from build123d import *

# Parameters (mm, degrees)
SKETCH1_W           = 38.354
SKETCH1_H           = 44.45
BOSS_EXTRUDE1_DEPTH = 25.4
SKETCH2_R           = 3.429
CUT_EXTRUDE1_DEPTH  = 44.45
SKETCH3_R           = 1.7272
CUT_EXTRUDE2_DEPTH  = 12.7
SKETCH5_R           = 1.7272
CUT_EXTRUDE4_DEPTH  = 12.7
SKETCH6_R           = 3.429
CUT_EXTRUDE5_DEPTH  = 38.354
SKETCH7_R           = 1.7272
CUT_EXTRUDE6_DEPTH  = 9.525
SKETCH11_W          = 38.354
SKETCH11_H          = 12.954
CUT_EXTRUDE9_DEPTH  = 3.2512
CUT_EXTRUDE7_START  = -7.62
SKETCH8_R           = 1.7272
CUT_EXTRUDE7_DEPTH  = 7.62
BOSS_EXTRUDE2_START = 2.54
SKETCH9_R           = 1.7272
SKETCH9_R_2         = 3.429
BOSS_EXTRUDE2_DEPTH = 2.54
SKETCH12_W          = 13.97
SKETCH12_H          = 25.4
CUT_EXTRUDE10_DEPTH = 3.2512
SKETCH13_R          = 1.7272
CUT_EXTRUDE11_DEPTH = 6.35
FILLET1_R           = 0.762


with BuildPart() as part:
    # Sketch1 → Boss-Extrude1 (new body)
    with BuildSketch(Plane(origin=(0, 0, 0), x_dir=(1, 0, 0), z_dir=(0, 1, 0))):
        with Locations((19.177, 22.225)):
            Rectangle(SKETCH1_W, SKETCH1_H)
    extrude(amount=BOSS_EXTRUDE1_DEPTH)

    # Sketch2 → Cut-Extrude1 (cut)
    with BuildSketch(Plane.XY):
        with Locations((22.479, 6.35)):
            Circle(SKETCH2_R)
    extrude(amount=-CUT_EXTRUDE1_DEPTH, mode=Mode.SUBTRACT)

    # Sketch3 → Cut-Extrude2 (cut)
    with BuildSketch(Plane(origin=(38.354, 0, 0), x_dir=(0, 0, -1), z_dir=(1, 0, 0))):
        with Locations((9.525, 12.7)):
            Circle(SKETCH3_R)
        with Locations((34.925, 12.7)):
            Circle(SKETCH3_R)
    extrude(amount=-CUT_EXTRUDE2_DEPTH, mode=Mode.SUBTRACT)

    # Sketch5 → Cut-Extrude4 (cut)
    with BuildSketch(Plane.ZY):
        with Locations((-31.75, 6.35)):
            Circle(SKETCH5_R)
        with Locations((-12.7, 6.35)):
            Circle(SKETCH5_R)
    extrude(amount=-CUT_EXTRUDE4_DEPTH, mode=Mode.SUBTRACT)

    # Sketch6 → Cut-Extrude5 (cut)
    with BuildSketch(Plane.ZY):
        with Locations((-22.225, 17.4625)):
            Circle(SKETCH6_R)
    extrude(amount=-CUT_EXTRUDE5_DEPTH, mode=Mode.SUBTRACT)

    # Sketch7 → Cut-Extrude6 (cut)
    with BuildSketch(Plane(origin=(0, 0, -44.45), x_dir=(-1, 0, 0), z_dir=(0, 0, -1))):
        with Locations((-31.0515, 6.35)):
            Circle(SKETCH7_R)
        with Locations((-13.9065, 6.35)):
            Circle(SKETCH7_R)
    extrude(amount=-CUT_EXTRUDE6_DEPTH, mode=Mode.SUBTRACT)

    # Sketch11 → Cut-Extrude9 (cut)
    with BuildSketch(Plane.XY):
        with Locations((19.177, 6.477)):
            Rectangle(SKETCH11_W, SKETCH11_H)
    extrude(amount=-CUT_EXTRUDE9_DEPTH, mode=Mode.SUBTRACT)

    # Sketch8 → Cut-Extrude7 (cut)
    with BuildSketch(Plane.XY.offset(-3.2512).offset(CUT_EXTRUDE7_START)):
        with Locations(Location((13.9065, 6.35, 0), (0, 0, 180))):
            Circle(SKETCH8_R)
        with Locations(Location((31.0515, 6.35, 0), (0, 0, 180))):
            Circle(SKETCH8_R)
    extrude(amount=CUT_EXTRUDE7_DEPTH, mode=Mode.SUBTRACT)

    # Sketch9 → Boss-Extrude2 (add)
    with BuildSketch(Plane(origin=(0, 0, -44.45), x_dir=(-1, 0, 0), z_dir=(0, 0, -1)).offset(BOSS_EXTRUDE2_START)):
        with BuildLine():
            Line((-32.545062003, 0), (-12.412937997, 0))
            ThreePointArc((-12.412937997, 0), (-22.479, 18.251600911), (-32.545062003, 0))
        make_face()
        with Locations(Location((-31.0515, 6.35, 0), (0, 0, 180))):
            Circle(SKETCH9_R, mode=Mode.SUBTRACT)
        with Locations(Location((-13.9065, 6.35, 0), (0, 0, 180))):
            Circle(SKETCH9_R, mode=Mode.SUBTRACT)
        with Locations(Location((-22.479, 6.35, 0), (0, 0, 180))):
            Circle(SKETCH9_R_2, mode=Mode.SUBTRACT)
    extrude(amount=-BOSS_EXTRUDE2_DEPTH)

    # Sketch12 → Cut-Extrude10 (cut)
    with BuildSketch(Plane(origin=(38.354, 0, 0), x_dir=(0, 0, -1), z_dir=(1, 0, 0))):
        with Locations((22.225, 12.7)):
            Rectangle(SKETCH12_W, SKETCH12_H)
    extrude(amount=-CUT_EXTRUDE10_DEPTH, mode=Mode.SUBTRACT)

    # Sketch13 → Cut-Extrude11 (cut)
    with BuildSketch(Plane(origin=(35.1028, 0, 0), x_dir=(0, 0, -1), z_dir=(1, 0, 0))):
        with Locations((22.225, 7.9375)):
            Circle(SKETCH13_R)
    extrude(amount=-CUT_EXTRUDE11_DEPTH, mode=Mode.SUBTRACT)

    # Fillet1
    fillet1_edges = [part.edges().sort_by_distance(p)[0] for p in [
        (38.354, 25.4, -7.62),
        (19.177, 25.4, -44.45),
        (0, 25.4, -22.225),
        (35.449531001, 0, -44.45),
        (38.354, 0, -9.2456),
        (19.177, 12.954, 0),
        (0, 6.477, -3.2512),
        (0, 12.954, -1.6256),
        (38.354, 6.477, -3.2512),
        (38.354, 12.954, -1.6256),
        (19.177, 0, -3.2512),
        (0, 0, -23.8506),
        (19.177, 25.4, 0),
        (6.206468999, 0, -44.45),
        (0, 12.7, -44.45),
        (38.354, 12.7, -44.45),
        (38.354, 19.177, 0),
        (12.412937997, 0, -45.72),
        (32.545062003, 0, -45.72),
        (0, 19.177, 0),
        (38.354, 25.4, -36.83),
        (38.354, 0, -36.83),
        (38.354, 12.7, -15.24),
        (38.354, 12.7, -29.21),
        (36.7284, 0, -15.24),
        (35.1028, 25.4, -22.225),
        (36.7284, 25.4, -15.24),
        (36.7284, 25.4, -29.21),
        (35.1028, 0, -22.225),
        (36.7284, 0, -29.21),
    ]]
    fillet(fillet1_edges, radius=FILLET1_R)


solid = part.part
Geometry check sheet. Reference: the model listing, model coordinates, mm. A direction names the side the tool comes from. Round coordinates to 2 decimals unless told otherwise and drop trailing zeros. Order: outer loops, then holes, each group sorted by start corner. A loop starts at its lowest first (then second) coordinate and runs counter-clockwise, first axis right, second up. Notation, with made-up numbers: M 6.25,88 L 16.25,88 A22 ccw 16.25,99 Z; hole C 30,-9 d11. An arc over 180 degrees is marked long. Answer in a Markdown table with one row per item. Add a question column.
Item 1: Sectioned sample at B-B, the plane x = 23.5. State how many separate pieces and enclosed holes the cut face has, plus the area to 3 significant figures.
Item 2: Depth check by flat-ended pin: pin 1 Ø2 at (x, y) = (31.05, 6.35) entering from +Z; pin 2 Ø11 at (y, z) = (17.46, -22.22) entering from +X; pin 3 Ø1.5 at (x, y) = (34, 6) entering from +Z. Enter the tip coordinate at first touch or a pass-through.
Item 3: Set-up check for faces 1 (the face through (19, 12.954, -2)), 2 (the face through (14, 6, -10.871)), 3 (the face through (14, 6, -34.925)), 4 (the face through (32.093, 11.014, -34.551)), 5 (the face through (36, 13, -15.24)): record each of +Z, -Z, +X, -X, +Y, -Y from which the full face is reachable in a straight line by a thin tool's end or side.
Item 4: Sectioned sample at A-A, the plane z = -31.75. Enter the section's corners in (x, y), plus the area to 3 significant figures.
Item 5: Material ranges on L1, parallel to X at y = 6.35, z = -45.25; L2, parallel to Y at x = 22.5, z = -22.5; L3, parallel to Y at x = 34.5, z = -35, recorded low to high. Write a range as [from, to].
Item 6: Draft check along Z on faces 6 (the face through (31.97, 9.65, -22)), 7 (the face through (19, 25.4, -23)), 8 (the face through (31, 6, -10.871)). Enter one of: released by +Z, released by -Z, zero draft, split by the parting line, or undercut.
Item 7: Sectioned sample at D-D, the plane y = 23.5. Enter the section's corners in (x, z).
Item 8: Sectioned sample at C-C, the plane z = -38.5. Enter the section's corners in (x, y), plus the area to 3 significant figures.
Filled in:
| question | item | result |
|---|---|---|
| 1 | separate pieces | 2 |
| 1 | enclosed holes | 1 |
| 1 | area | 809 mm² |
| 2 | pin 1 | stops at z = -10.87 |
| 2 | pin 2 | stops at x = 35.1 |
| 2 | pin 3 | stops at z = -3.25 |
| 3 | face 1 | +Z, +X, -X, -Y |
| 3 | face 2 | +Z |
| 3 | face 3 | -Z |
| 3 | face 4 | +X |
| 3 | face 5 | +X, +Y, -Y |
| 4 | outline | M 0,0.76 A0.76 ccw 0.76,0 L 37.59,0 A0.76 ccw 38.35,0.76 L 38.35,24.64 A0.76 ccw 37.59,25.4 L 0.76,25.4 A0.76 ccw 0,24.64 L 0,8.08 L 12.7,8.08 L 12.7,4.62 L 0,4.62 Z; hole C 22.48,6.35 d6.86 |
| 4 | area | 893 mm² |
| 5 | L1 | x = [10.58, 12.18], [15.63, 19.05], [25.91, 29.32], [32.78, 34.38] |
| 5 | L2 | y = [0, 2.92], [9.78, 14.04], [20.88, 25.4] |
| 5 | L3 | y = [0, 10.97], [14.43, 25.4] |
| 6 | face 6 | undercut |
| 6 | face 7 | zero draft |
| 6 | face 8 | released by +Z |
| 7 | outline | M 0,-43.69 A0.76 ccw 0.76,-44.45 L 37.59,-44.45 A0.76 ccw 38.35,-43.69 L 38.35,-29.97 A0.76 ccw 37.59,-29.21 L 35.1,-29.21 L 35.1,-15.24 L 37.59,-15.24 A0.76 ccw 38.35,-14.48 L 38.35,-0.76 A0.76 ccw 37.59,0 L 0.76,0 A0.76 ccw 0,-0.76 Z |
| 8 | outline | M 0,0.76 A0.76 ccw 0.76,0 L 37.59,0 A0.76 ccw 38.35,0.76 L 38.35,24.64 A0.76 ccw 37.59,25.4 L 0.76,25.4 A0.76 ccw 0,24.64 Z; hole C 13.91,6.35 d3.45; hole C 22.48,6.35 d6.86; hole C 31.05,6.35 d3.45 |
| 8 | area | 918 mm² |
